```python
from build123d import *

# Parameters (mm, degrees)
F1_DEPTH = 12.7
F2_R     = 1.27


with BuildPart() as f1:
    # F0 (on Front) → F1 (new body)
    with BuildSketch(Plane.XZ):
        with BuildLine():
            Line((-60.66708, 18.066773), (-60.66708, 68.866773))
            Line((-60.66708, 68.866773), (-63.84208, 68.866773))
            Line((-63.84208, 68.866773), (-63.84208, 18.066773))
            ThreePointArc((-63.84208, 18.066773), (-51.14208, 5.366773), (-38.44208, 18.066773))
            Line((-38.44208, 18.066773), (-41.61708, 18.066773))
            ThreePointArc((-41.61708, 18.066773), (-51.14208, 8.541773), (-60.66708, 18.066773))
        make_face()
    extrude(amount=F1_DEPTH)

    # F2
    f2_edges = [f1.edges().sort_by_distance(p)[0] for p in [
        (-60.66708, -12.7, 43.466773),
        (-60.66708, 0, 43.466773),
        (-38.44208, -6.35, 18.066773),
        (-41.61708, -6.35, 18.066773),
        (-60.66708, -6.35, 68.866773),
    ]]
    fillet(f2_edges, radius=F2_R)


solid = f1.part
```
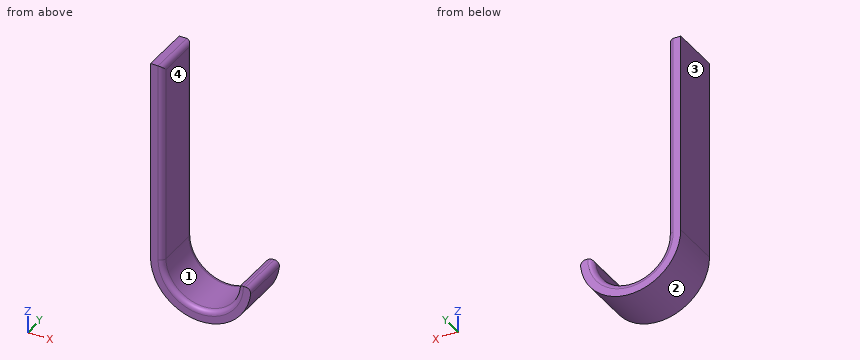
Work out the finished part from the listing and answer in its coordinate system (mm). Face numbers are marked on the shaded views. Coordinates: 2 decimals unless noted, no trailing zeros. Loops run counter-clockwise (first coordinate to the right, second up) from the corner with the lowest first, then second, coordinate; pieces in that order, holes last.
1) Section B-B (z = 46.5) is taken. Give the vertices of the cut face in (x, y).
Results:
outline: (-63.84, -12.7) - (-61.94, -12.7) arc R1.27 ccw to (-60.67, -11.43) - (-60.67, -1.27) arc R1.27 ccw to (-61.94, 0) - (-63.84, 0) - close
2) Consider probe 1 along X at (y, z) = (-3.5, 45); probe 2 along Z at (x, y) = (-51.5, -5.75); probe 3 along X at (y, z) = (-12, 12). Determine where each line is inside the solid, lowest interval first.
Results:
probe 1: x = -63.84 to -60.67
probe 2: z = 5.37 to 8.55
probe 3: x = -62.3 to -58.66, -43.62 to -39.98
3) For a pull along X with two mould halves and no side action, classify the marked faces 1, 2, 3 and 4 as +X half, -X half, draft (parallel to the pull), parting line (faces both ways), or undercut.
Results:
face 1: undercut
face 2: parting line
face 3: -X half
face 4: +X half
4) Flat-ended cylindrical pins translate along their axes: pin 1 (3 mm diameter, centred on x = -60.5, y = -6, fed in from -Z); pin 2 (4 mm diameter, centred on y = -1.5, z = 28.5, fed in from +X); pin 3 (2 mm diameter, centred on x = -44.5, y = -5, fed in from -Z). Find the tip coordinate at first contact, or state that the pin passes through.
Results:
pin 1: stops at z = 8.09
pin 2: stops at x = -60.67
pin 3: stops at z = 6.69
5) Section A-A (y = -9) is taken. Give the vertices of the cut face in (x, z) (3 decimals), plus the area to 3 significant figures.
Results:
outline: (-63.842, 18.067) arc R12.7 ccw to (-38.521, 16.656) arc R1.27 ccw to (-39.783, 18.067) - (-40.422, 18.067) arc R1.27 ccw to (-41.683, 16.946) arc R9.525 cw to (-60.667, 18.067) - (-60.667, 67.597) arc R1.27 ccw to (-61.937, 68.867) - (-63.842, 68.867) - close
area: 271 mm2
